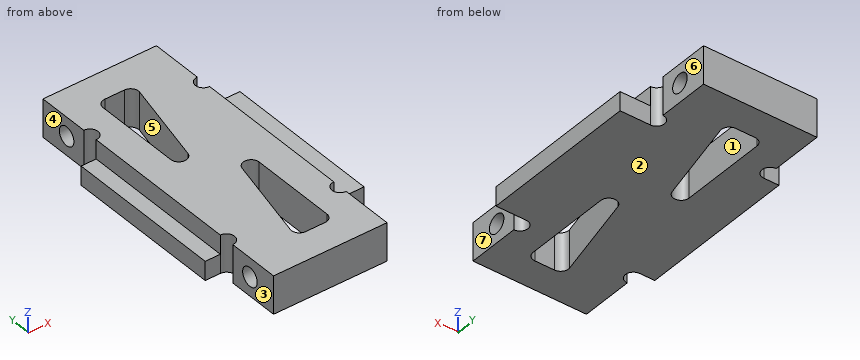
Autodesk Inventor part; units mm, degrees
ref_plane "YZ Plane" through (0, 0, 0) normal (1, 0, 0) x (0, 1, 0)
ref_plane "XZ Plane" through (0, 0, 0) normal (0, 1, 0) x (-1, 0, 0)
ref_plane "XY Plane" through (0, 0, 0) normal (0, 0, 1) x (1, 0, 0)
sketch "スケッチ1" plane through (0, 0, 0) normal (0, 0, 1) x (1, 0, 0)
  line L0 (-7.5, -19.5) -> (7.5, -19.5) construction
  line L1 (7.5, -19.5) -> (7.5, 19.5) construction
  line L2 (7.5, 19.5) -> (-7.5, 19.5) construction
  line L3 (-7.5, 19.5) -> (-7.5, -19.5) construction
  line L4 (-7.5, -19.5) -> (7.5, 19.5) construction
  line L5 (7.5, -19.5) -> (-7.5, 19.5) construction
  line L6 (-7.5, 10.5) -> (-7.5, 19.5) construction
  line L7 (-7.5, 19.5) -> (7.5, 19.5)
  line L8 (7.5, 19.5) -> (7.5, 10.5) construction
  line L9 (-7.5, 10.5) -> (-9.5, 10.5)
  line L10 (-9.5, 10.5) -> (-9.5, -10.5)
  line L11 (-9.5, -10.5) -> (-7.5, -10.5)
  line L12 (-7.5, -10.5) -> (-7.5, -19.5) construction
  line L13 (-7.5, -19.5) -> (7.5, -19.5)
  line L14 (7.5, -19.5) -> (7.5, -10.5) construction
  line L15 (7.5, -10.5) -> (11.5, -10.5)
  line L16 (11.5, -10.5) -> (11.5, 10.5)
  line L17 (11.5, 10.5) -> (7.5, 10.5)
  line L18 (0, 0) -> (11.5, 0) construction
  circle A0 centre (-7.5, 11.55) radius 1.05 construction
  circle A1 centre (-7.5, -11.55) radius 1.05 construction
  circle A2 centre (7.5, 11.55) radius 1.05 construction
  circle A3 centre (7.5, -11.55) radius 1.05 construction
  line L19 (-7.5, 19.5) -> (-7.5, 12.6)
  arc A4 (-7.5, 10.5) -> (-7.5, 12.6) centre (-7.5, 11.55) ccw
  arc A5 (-7.5, -12.6) -> (-7.5, -10.5) centre (-7.5, -11.55) ccw
  line L20 (-7.5, -12.6) -> (-7.5, -19.5)
  line L21 (7.5, 12.6) -> (7.5, 19.5)
  arc A6 (7.5, 12.6) -> (7.5, 10.5) centre (7.5, 11.55) ccw
  line L22 (7.5, -12.6) -> (7.5, -19.5)
  arc A7 (7.5, -10.5) -> (7.5, -12.6) centre (7.5, -11.55) ccw
  dimension "d21" = 2
  dimension "d23" = 4
  dimension "d30" = 15
  dimension "d48" = 9
  dimension "d49" = 39
  dimension "d50" = 2.1
extrude "押し出し1" add sketch "スケッチ1" along normal blind 5
sketch "スケッチ2" plane through (7.5, -19.5, 0) normal (1, 0, 0) x (0, 0, -1)
  line L0 (0, 0) -> (-5, 0)
  line L1 (0, 39) -> (-5, 39)
  point P0 (0, 19.5)
  point P1 (-2.5, 4)
  point P2 (-2.5, 35)
  point P3 (-2.5, 0)
  dimension "d53" = 4
  dimension "d54" = 4
hole "穴1" at (7.5, -15.5, 2.5) at (7.5, 15.5, 2.5) direction (-1, 0, 0) diameter 2.459 depth 2.5 tip angle 118
mirror "ミラー1" about plane through (0, 0, 0) normal (1, 0, 0) of "穴1"
sketch "スケッチ3" plane through (0, 0, 5) normal (0, 0, 1) x (1, 0, 0)
  line L0 (7.5, 12.6) -> (7.5, 19.5)
  line L1 (-7.5, 19.5) -> (-7.5, 12.6)
  line L2 (-12.0807, 15.6684) -> (-7.5, 15.6684)
  line L3 (-7.5, 15.6684) -> (-7.5, -16.7148)
  line L4 (-7.5, -16.7148) -> (-12.0807, -16.7148)
  line L5 (-12.0807, -16.7148) -> (-12.0807, 15.6684)
  line L6 (12.9714, 11.55) -> (7.5, 11.55)
  line L7 (7.5, 11.55) -> (7.5, -15.9078)
  line L8 (7.5, -15.9078) -> (12.9714, -15.9078)
  line L9 (12.9714, -15.9078) -> (12.9714, 11.55)
  point P0 (0, 0)
extrude "押し出し2" cut sketch "スケッチ3" against normal blind 2.5
sketch "スケッチ4" plane through (0, 0, 5) normal (0, 0, 1) x (1, 0, 0)
  line L0 (7.5, 12.6) -> (7.5, 19.5)
  line L1 (7.5, 19.5) -> (-7.5, 19.5)
  line L2 (-7.5, -12.6) -> (-7.5, -19.5)
  line L3 (-7.5, -19.5) -> (7.5, -19.5)
  line L4 (-3.5, 15.5) -> (3.5, 15.5) construction
  line L5 (3.5, 15.5) -> (3.5, -15.5) construction
  line L6 (3.5, -15.5) -> (-3.5, -15.5) construction
  line L7 (-3.5, -15.5) -> (-3.5, 15.5) construction
  line L8 (3.5, 15.5) -> (-3.5, -15.5) construction
  line L9 (1.4496, 15.5) -> (-3.5, 15.5)
  line L10 (-3.5, 15.5) -> (-3.5, -6.4199)
  line L11 (-3.5, -6.4199) -> (1.4496, 15.5)
  line L12 (-1.4496, -15.5) -> (3.5, -15.5)
  line L13 (3.5, -15.5) -> (3.5, 6.4199)
  line L14 (3.5, 6.4199) -> (-1.4496, -15.5)
  point P0 (0, 0)
  dimension "d64" = 4
  dimension "d65" = 4
  dimension "d66" = 4
  dimension "d67" = 4
  dimension "d68" = 4
extrude "押し出し3" cut sketch "スケッチ4" against normal blind 5
fillet "フィレット1" radius 1.05 6 edges at (-1.4496, -15.5, 2.5) (-3.5, 15.5, 2.5) (1.4496, 15.5, 2.5) (3.5, 6.4199, 2.5) (-3.5, -6.4199, 2.5) (3.5, -15.5, 2.5)
equation "\"d48\" = d26 + d35"
equation "\"d49\" = d38"
equation "\"d66\" = d65"
equation "\"d68\" = d67"
equation "\"d26\" = 5"
equation "\"d35\" = 4"
equation "\"d38\" = 39"
properties part number "Trunk_armpit_frame" material "アセタール樹脂、黒"
The model under review builds one solid part; all positions refer to its coordinate system, in mm. Face numbers are marked on the shaded views. A direction names the side the tool comes from. Coordinates: 2 decimals unless noted, no trailing zeros. Loops run counter-clockwise (first coordinate to the right, second up) from the corner with the lowest first, then second, coordinate; pieces in that order, holes last.
(1) Consider section B-B, the plane y = 13.5. Give the boundary of the cut face in (x, z), plus the area to 3 significant figures.
Determined:
outline: (-7.5, 0) - (-3.5, 0) - (-3.5, 5) - (-7.5, 5) - close; (1, 0) - (7.5, 0) - (7.5, 5) - (1, 5) - close
area: 52.5 mm2
(2) Consider section D-D, the plane x = -0.75. Give the boundary of the cut face in (y, z).
Determined:
outline: (-19.5, 0) - (-15.3, 0) - (-15.3, 5) - (-19.5, 5) - close; (-12.4, 0) - (5.76, 0) - (5.76, 5) - (-12.4, 5) - close; (15.5, 0) - (19.5, 0) - (19.5, 5) - (15.5, 5) - close
(3) Tool access review of the marked faces 4, 5, 6 and 7: name each direction out of +Z, -Z, +X, -X, +Y, -Y from which nothing blocks a thin tool from reaching the whole face with its end or side.
Determined:
face 4: +Z, -Z, -X, +Y
face 5: +Z, -Z
face 6: +Z, -Z, +X, +Y
face 7: +Z, -Z, +X, -Y
(4) Consider section C-C, the plane x = -5.75. Give the boundary of the cut face in (y, z), plus the area to 3 significant figures.
Determined:
outline: (-19.5, 0) - (19.5, 0) - (19.5, 5) - (-19.5, 5) - close; hole circle Ø2.46 at (-15.5, 2.5); hole circle Ø2.46 at (15.5, 2.5)
area: 186 mm2
(5) Consider section A-A, the plane y = 1. Give the boundary of the cut face in (x, z), plus the area to 3 significant figures.
Determined:
outline: (-9.5, 0) - (11.5, 0) - (11.5, 2.5) - (7.5, 2.5) - (7.5, 5) - (-7.5, 5) - (-7.5, 2.5) - (-9.5, 2.5) - close
area: 90.0 mm2
(6) Wall thickness on L1, parallel to Y at x = 5.7, z = 2.5; L2, parallel to Z at x = 5.65, y = -15.5; L3, parallel to X at y = -14.5, z = 3.8: over which ranges is each line inside the solid? List them lowest first.
Determined:
L1: y = -19.5 to -16.73, -14.27 to 14.27, 16.73 to 19.5
L2: z = 0 to 1.27, 3.73 to 5
L3: x = -7.5 to -1.18, 3.5 to 7.5
(7) Insertion check: P1, Ø5, axis at x = -2, y = -3, coming from the -Z side; P2, Ø0.8, axis at y = 4.5, z = 4, coming from the +X side; P3, Ø1.2, axis at y = -3.5, z = 3.5, coming from the -X side; P4, Ø1.2, axis at x = 10, z = 1, coming from the -Y side. Each pin has a flat end and moves straight along its axis. Give the tip position at first contact, or say it passes through.
Determined:
P1: stops at z = 0
P2: stops at x = 7.5
P3: stops at x = -7.5
P4: stops at y = -10.5
(8) Draft analysis for pull direction X (two halves, no side actions). For the marked faces 1, 2 and 3, state which applies: +X half, -X half, draft (parallel to the pull), parting line (faces both ways), or undercut.
Determined:
face 1: undercut
face 2: draft
face 3: -X half
